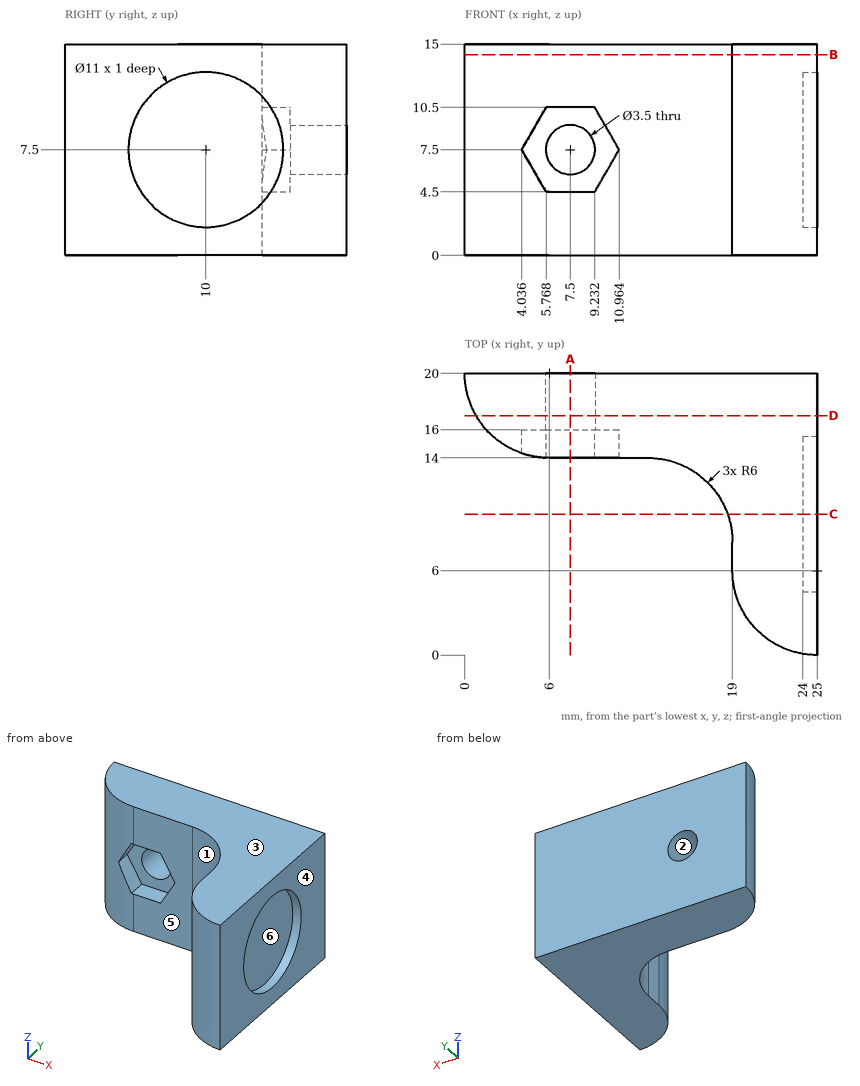
Input: dimensioned drawing with shaded views. Units: mm. Origin: part minimum x, y, z. A direction names the side the tool comes from. Coordinates: 2 decimals unless noted, no trailing zeros. Order: outer loops, then holes, each group sorted by start corner. A loop starts at its lowest first (then second) coordinate and runs counter-clockwise, first axis right, second up.
Item 1: Section query C-C (y = 10). Output: boundary loops of the cut face in (x, z).
Answer:
outline: (18.66, 0) - (25, 0) - (25, 2) - (24, 2) - (24, 13) - (25, 13) - (25, 15) - (18.66, 15) - close
Item 2: Access query for the marked faces 4, 5 and 6. Directions: +Z, -Z, +X, -X, +Y, -Y. A direction counts if a zero-diameter tool reaches every point of the face in a straight line with its end or side. Return the directions, or none.
Answer:
face 4: +Z, -Z, +X, +Y, -Y
face 5: +Z, -Z, -X, -Y
face 6: +X
Item 3: Section query A-A (x = 7.5). Output: boundary loops of the cut face in (y, z), then the cut area to 3 significant figures.
Answer:
outline: (14, 0) - (20, 0) - (20, 5.75) - (16, 5.75) - (16, 4.5) - (14, 4.5) - close; (14, 10.5) - (16, 10.5) - (16, 9.25) - (20, 9.25) - (20, 15) - (14, 15) - close
area: 64.0 mm2
Item 4: Section query B-B (z = 14.25). Output: boundary loops of the cut face in (x, y).
Answer:
outline: (0, 20) arc R6 ccw to (6, 14) - (13, 14) arc R6 cw to (19, 8) - (19, 6) arc R6 ccw to (25, 0) - (25, 20) - close
Item 5: Material intervals for line 1 along Z through (x, y) = (24.35, 10); line 2 along Z through (x, y) = (7.5, 18); line 3 along Y through (x, z) = (11.5, 5), sorted ascending.
Answer:
line 1: z = 0 to 2, 13 to 15
line 2: z = 0 to 5.75, 9.25 to 15
line 3: y = 14 to 20
Item 6: Section query D-D (y = 17). Output: boundary loops of the cut face in (x, z).
Answer:
outline: (0.8, 0) - (25, 0) - (25, 15) - (0.8, 15) - close; hole circle Ø3.5 at (7.5, 7.5)
Item 7: Draft query along Z for the marked faces 1, 2 and 3. Return one class per face: released by +Z, released by -Z, zero draft, split by the parting line, or undercut.
Answer:
face 1: zero draft
face 2: undercut
face 3: released by +Z
Item 8: Contact query for flat-ended pins moving along their axis: P1, Ø3.5, axis at y = 11, z = 9, coming from the +X side; P2, Ø5.5, axis at x = 9.5, z = 10, coming from the -Y side; P3, Ø1, axis at y = 7, z = 6.5, coming from the -X side; P4, Ø3, axis at x = 7.5, z = 7.5, coming from the +Y side. Output: stop coordinate, or through.
Answer:
P1: stops at x = 24
P2: stops at y = 14
P3: stops at x = 19
P4: passes through
